from build123d import *

# Parameters (mm, degrees)
F0_R     = 2.5
F1_DEPTH = 5
F2_R     = 10
F3_R     = 1


with BuildPart() as f1:
    # F0 (on Top) → F1 (new body)
    with BuildSketch(Plane.XY):
        with BuildLine():
            ThreePointArc((-2.3070607836, 0), (-2.4774316521, 1.2940952255), (-2.9769337647, 2.5))
            ThreePointArc((-2.9769337647, 2.5), (-12.3070607836, 0), (-2.9769337647, -2.5))
            ThreePointArc((-2.9769337647, -2.5), (-2.4774316521, -1.2940952255), (-2.3070607836, 0))
        make_face()
        with Locations((-7.3070607836, 0)):
            Circle(F0_R, mode=Mode.SUBTRACT)
        with BuildLine():
            ThreePointArc((38.3628121975, -2.5), (37.6929392164, 0), (38.3628121975, 2.5))
            Line((38.3628121975, 2.5), (-2.9769337647, 2.5))
            ThreePointArc((-2.9769337647, 2.5), (-2.4774316521, 1.2940952255), (-2.3070607836, 0))
            ThreePointArc((-2.3070607836, 0), (-2.4774316521, -1.2940952255), (-2.9769337647, -2.5))
            Line((-2.9769337647, -2.5), (38.3628121975, -2.5))
        make_face()
        with BuildLine():
            ThreePointArc((38.3628121975, -2.5), (43.9870344419, -4.8296291314), (47.6929392164, 0))
            ThreePointArc((47.6929392164, 0), (43.9870344419, 4.8296291314), (38.3628121975, 2.5))
            ThreePointArc((38.3628121975, 2.5), (37.6929392164, 0), (38.3628121975, -2.5))
        make_face()
        with Locations((42.6929392164, 0)):
            Circle(F0_R, mode=Mode.SUBTRACT)
    extrude(amount=F1_DEPTH)

    # F2
    f2_edges = [f1.edges().sort_by_distance(p)[0] for p in [
        (-2.976934, 2.5, 2.5),
        (-2.976934, -2.5, 2.5),
        (38.362812, -2.5, 2.5),
        (38.362812, 2.5, 2.5),
    ]]
    fillet(f2_edges, radius=F2_R)

    # F3
    f3_edges = [f1.edges().sort_by_distance(p)[0] for p in [
        (17.692939, 2.5, 5),
        (-1.90225, 2.925729, 5),
        (17.692939, 2.5, 0),
    ]]
    fillet(f3_edges, radius=F3_R)


solid = f1.part
Geometry check sheet. Reference: the model listing, model coordinates, mm. A direction names the side the tool comes from. Round coordinates to 2 decimals unless told otherwise and drop trailing zeros. Order: outer loops, then holes, each group sorted by start corner. A loop starts at its lowest first (then second) coordinate and runs counter-clockwise, first axis right, second up. Notation, with made-up numbers: M 18.25,76 L 51.25,76 A9 cw 51.25,83 Z; hole C 50,-37.75 d8. An arc over 180 degrees is marked long. Answer in a Markdown table with one row per item. Add a question column.
Item 1: Sectioned sample at B-B, the plane x = 20.5. Enter the section's corners in (y, z), plus the area to 3 significant figures.
Item 2: Sectioned sample at C-C, the plane z = 4.5. Enter the section's corners in (x, y).
Item 3: Set-up check for faces 1 (the face through (-1.941, -2.938, 2.521)), 2 (the face through (17.927, -2.199, 4.715)), 3 (the face through (17.459, 2.199, 0.285)), 4 (the face through (17.927, -2.199, 0.285)), 5 (the face through (17.459, 2.199, 4.715)): record each of +Z, -Z, +X, -X, +Y, -Y from which the full face is reachable in a straight line by a thin tool's end or side.
Item 4: Material ranges on L1, parallel to X at y = -1.5, z = 3.5; L2, parallel to X at y = -1, z = 0.9; L3, parallel to Y at x = 6, z = 1.9, recorded low to high. Write a range as [from, to].
Item 5: Sectioned sample at A-A, the plane z = 1.55. Enter the section's corners in (x, y), plus the area to 3 significant figures.
Item 6: Depth check by flat-ended pin: pin 1 Ø1 at (y, z) = (3, 3) entering from -X; pin 2 Ø1.5 at (x, z) = (14, 2.5) entering from -Y; pin 3 Ø4.5 at (x, y) = (-7.31, 0) entering from -Z. Enter the tip coordinate at first touch or a pass-through.
Filled in:
| question | item | result |
|---|---|---|
| 1 | outline | M -2.5,1 A1 ccw -1.5,0 L 1.5,0 A1 ccw 2.5,1 L 2.5,4 A1 ccw 1.5,5 L -1.5,5 A1 ccw -2.5,4 Z |
| 1 | area | 24.1 mm² |
| 2 | outline | M -4.62,-4.06 A10.13 cw 0.98,-2.37 L 34.4,-2.37 A10.13 cw 40,-4.06 A4.87 ccw long 40,4.06 A10.13 cw 34.4,2.37 L 0.98,2.37 A10.13 cw -4.62,4.06 A4.87 ccw long Z; hole C -7.31,0 d5; hole C 42.69,0 d5 |
| 3 | face 1 | +Z, -Z, -Y |
| 3 | face 2 | +Z, -Y |
| 3 | face 3 | -Z, +Y |
| 3 | face 4 | -Z, -Y |
| 3 | face 5 | +Z, +Y |
| 4 | L1 | x = [-12.08, -9.31], [-5.31, 40.69], [44.69, 47.46] |
| 4 | L2 | x = [-12.2, -9.6], [-5.02, 40.4], [44.98, 47.59] |
| 4 | L3 | y = [-2.5, 2.5] |
| 5 | outline | M -4.54,-4.17 A10 cw 0.98,-2.5 L 34.4,-2.5 A10 cw 39.93,-4.17 A5 ccw long 39.93,4.17 A10 cw 34.4,2.5 L 0.98,2.5 A10 cw -4.54,4.17 A5 ccw long Z; hole C -7.31,0 d5; hole C 42.69,0 d5 |
| 5 | area | 326 mm² |
| 6 | pin 1 | stops at x = -11.64 |
| 6 | pin 2 | stops at y = -2.5 |
| 6 | pin 3 | passes through |
